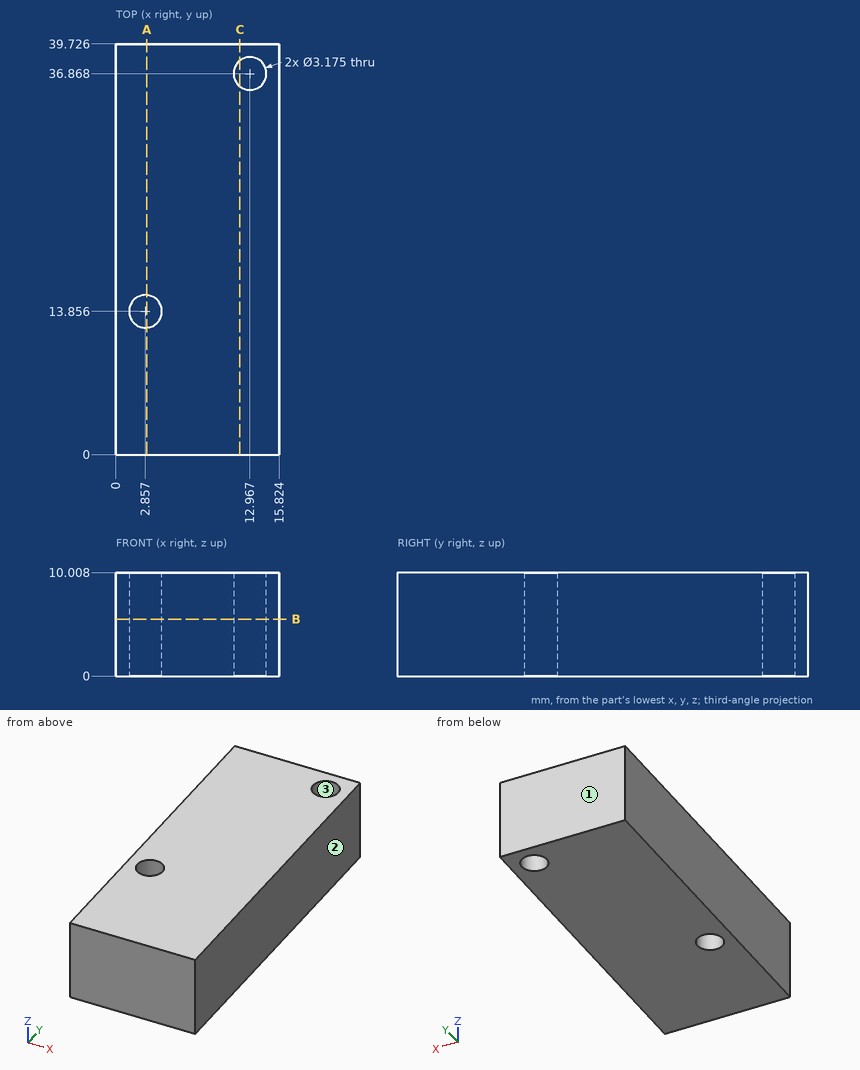
Can you work these out from the drawing? Everything is in mm from the part's minimum corner. Give positions to 0.01 mm unless a question says otherwise; leave off trailing zeros. Order: outer loops, then holes, each group sorted by start corner. A loop starts at its lowest first (then second) coordinate and runs counter-clockwise, first axis right, second up.
Item 1: I need wall thicknesses on line 1 (Y direction, x = 3, z = 9.5) (1 decimal); line 2 (X direction, y = 37, z = 9.75) (1 decimal); line 3 (Y direction, x = 4.25, z = 4.25) (1 decimal). Which ranges of each line are inside material? Lowest first, please.
Item 2: I'm going to push a flat-ended pin straight in: pin 1 (5 mm diameter, centred on y = 20, z = 8.5, fed in from -X). Where does the tip first touch, or does it pass through?
Item 3: If we section it at C-C, the plane x = 12: Write out the boundary of the cut face in (y, z) (1 decimal).
Item 4: If we section it at A-A, the plane x = 3: Write out the boundary of the cut face in (y, z) (1 decimal).
Item 5: If we mould it in two halves opening along X, with no side actions, what happens to the marked faces 1, 2 and 3? For each: pulls with the +X half, pulls with the -X half, needs draft (parallel to the pull), parting line crosses it, or undercut.
Item 6: If we section it at B-B, the plane z = 5.5: Write out the boundary of the cut face in (x, y) (1 decimal), plus the area to 3 significant figures.
Values:
1. line 1: y = 0 to 12.3, 15.4 to 39.7
1. line 2: x = 0 to 11.4, 14.5 to 15.8
1. line 3: y = 0 to 13.1, 14.6 to 39.7
2. pin 1: stops at x = 0
3. outline: (0, 0) - (35.6, 0) - (35.6, 10) - (0, 10) - close; (38.1, 0) - (39.7, 0) - (39.7, 10) - (38.1, 10) - close
4. outline: (0, 0) - (12.3, 0) - (12.3, 10) - (0, 10) - close; (15.4, 0) - (39.7, 0) - (39.7, 10) - (15.4, 10) - close
5. face 1: needs draft
5. face 2: pulls with the +X half
5. face 3: undercut
6. outline: (0, 0) - (15.8, 0) - (15.8, 39.7) - (0, 39.7) - close; hole circle Ø3.2 at (2.9, 13.9); hole circle Ø3.2 at (13, 36.9)
6. area: 613 mm2
